from build123d import *

# Parameters (mm, degrees)
EXTRUDE_DEPTH     = 20
BOX003_W          = 15
BOX003_H          = 7.5
BOX003_DEPTH      = 6
CYLINDER003_R     = 2.1
CYLINDER003_DEPTH = 5
CYLINDER002_R     = 1.05
CYLINDER002_DEPTH = 7
BOX002_W          = 13
BOX002_H          = 13
BOX002_DEPTH      = 6
CYLINDER001_R     = 2.65
CYLINDER001_DEPTH = 5
CYLINDER_R        = 5.2
CYLINDER_DEPTH    = 20
BOX001_W          = 20.5
BOX001_H          = 20.5
BOX001_DEPTH      = 25
BOX004_W          = 7.5
BOX004_H          = 13
BOX004_DEPTH      = 6
BOX_W             = 40.5
BOX_H             = 62.8
BOX_DEPTH         = 25
FILLET_1_R        = 3
FILLET_2_R        = 1


with BuildPart() as obj1:
    # Sketch → Extrude (new body)
    with BuildSketch(Plane.YZ):
        with BuildLine():
            ThreePointArc((-3.606243, 3.606246), (0, -5.1), (3.606243, 3.606246))
            Line((2.112489, 5.1), (3.606243, 3.606246))
            Line((-2.112489, 5.1), (2.112489, 5.1))
            Line((-3.606243, 3.606246), (-2.112489, 5.1))
        make_face()
    extrude(amount=EXTRUDE_DEPTH)


with BuildPart() as obj1_1:
    # Extrude placement: moved
    add(obj1.part.moved(Location((20.5, 41.65, 15))))


with BuildPart() as hueco_taladro4:
    # Box003 → Box003 (new body)
    with BuildSketch(Plane(origin=(0, 39, 14), x_dir=(1, 0, 0), z_dir=(0, 0, 1))):
        with Locations((7.5, 3.75)):
            Rectangle(BOX003_W, BOX003_H)
    extrude(amount=BOX003_DEPTH)


with BuildPart() as taladro4:
    # Cylinder003 → Cylinder003 (new body)
    with BuildSketch(Plane(origin=(10, 42.7, 20), x_dir=(1, 0, 0), z_dir=(0, 0, 1))):
        Circle(CYLINDER003_R)
    extrude(amount=CYLINDER003_DEPTH)


with BuildPart() as clone005:
    # Clone005 base: copy of taladro4
    add(taladro4.part)


with BuildPart() as clone005_1:
    # Clone005 placement: moved
    add(clone005.part.moved(Location((15.5, 13.1, 0))))


with BuildPart() as taladro_endstop:
    # Cylinder002 → Cylinder002 (new body)
    with BuildSketch(Plane(origin=(35.5, 26.14, 12), x_dir=(1, 0, 0), z_dir=(0, 0, 1))):
        Circle(CYLINDER002_R)
    extrude(amount=CYLINDER002_DEPTH)


with BuildPart() as clone004:
    # Clone004 base: copy of taladro_endstop
    add(taladro_endstop.part)


with BuildPart() as clone004_1:
    # Clone004 placement: moved
    add(clone004.part.moved(Location((0, 7, 0))))


with BuildPart() as hueco_endstop:
    # Box002 → Box002 (new body)
    with BuildSketch(Plane(origin=(27.5, 23.14, 19), x_dir=(1, 0, 0), z_dir=(0, 0, 1))):
        with Locations((6.5, 6.5)):
            Rectangle(BOX002_W, BOX002_H)
    extrude(amount=BOX002_DEPTH)


with BuildPart() as taladro5:
    # Cylinder001 → Cylinder001 (new body)
    with BuildSketch(Plane(origin=(30.5, 10, 0), x_dir=(1, 0, 0), z_dir=(0, 0, 1))):
        Circle(CYLINDER001_R)
    extrude(amount=CYLINDER001_DEPTH)


with BuildPart() as clone002:
    # Clone002 base: copy of taladro5
    add(taladro5.part)


with BuildPart() as clone002_1:
    # Clone002 placement: moved
    add(clone002.part.moved(Location((-20.5, 21, 0))))


with BuildPart() as clone003:
    # Clone003 base: copy of Clone002
    add(clone002_1.part)


with BuildPart() as clone003_1:
    # Clone003 placement: moved
    add(clone003.part.moved(Location((0, 21.3, 0))))


with BuildPart() as taladro10:
    # Cylinder → Cylinder (new body)
    with BuildSketch(Plane(origin=(30.5, 10, 5), x_dir=(1, 0, 0), z_dir=(0, 0, 1))):
        Circle(CYLINDER_R)
    extrude(amount=CYLINDER_DEPTH)


with BuildPart() as clone:
    # Clone base: copy of taladro10
    add(taladro10.part)


with BuildPart() as clone_1:
    # Clone placement: moved
    add(clone.part.moved(Location((-20.5, 21, 0))))


with BuildPart() as clone001:
    # Clone001 base: copy of Clone
    add(clone_1.part)


with BuildPart() as clone001_1:
    # Clone001 placement: moved
    add(clone001.part.moved(Location((0, 21.3, 0))))


with BuildPart() as obj2:
    # Box001 → Box001 (new body)
    with BuildSketch(Plane.XY):
        with Locations((10.25, 10.25)):
            Rectangle(BOX001_W, BOX001_H)
    extrude(amount=BOX001_DEPTH)


with BuildPart() as huecos:
    # Box004 → Box004 (new body)
    with BuildSketch(Plane(origin=(21.75, 49.8, 14), x_dir=(1, 0, 0), z_dir=(0, 0, 1))):
        with Locations((3.75, 6.5)):
            Rectangle(BOX004_W, BOX004_H)
    extrude(amount=BOX004_DEPTH)

    # Fusion: union hueco_taladro4, Clone005, taladro4, Clone004, taladro_endstop, hueco_endstop, Clone003, Clone002, taladro5, Clone001, Clone, taladro10, obj2
    add(hueco_taladro4.part)
    add(clone005_1.part)
    add(taladro4.part)
    add(clone004_1.part)
    add(taladro_endstop.part)
    add(hueco_endstop.part)
    add(clone003_1.part)
    add(clone002_1.part)
    add(taladro5.part)
    add(clone001_1.part)
    add(clone_1.part)
    add(taladro10.part)
    add(obj2.part)


with BuildPart() as obj3:
    # Box → Box (new body)
    with BuildSketch(Plane.XY):
        with Locations((20.25, 31.4)):
            Rectangle(BOX_W, BOX_H)
    extrude(amount=BOX_DEPTH)

    # Cut: cut huecos
    add(huecos.part, mode=Mode.SUBTRACT)

    # Cut001: cut obj1
    add(obj1_1.part, mode=Mode.SUBTRACT)

    # Fillet 1
    fillet_1_edges = [obj3.edges().sort_by_distance(p)[0] for p in [
        (0, 62.8, 12.5),
        (40.5, 62.8, 12.5),
        (40.5, 0, 12.5),
    ]]
    fillet(fillet_1_edges, radius=FILLET_1_R)

    # Fillet 2
    fillet_2_edges = [obj3.edges().sort_by_distance(p)[0] for p in [
        (0, 20.5, 12.5),
        (20.5, 0, 12.5),
    ]]
    fillet(fillet_2_edges, radius=FILLET_2_R)


with BuildPart() as obj4:
    # Part__Mirroring: instance of obj3
    add(obj3.part.mirror(Plane(origin=(0, 0, 0), x_dir=(1, 0, 0), z_dir=(0, 1, 0))))


solid = obj4.part
The model under review builds one solid part; all positions refer to its coordinate system, in mm. A direction names the side the tool comes from. Round coordinates to 2 decimals unless told otherwise and drop trailing zeros. Write each loop counter-clockwise with the first axis right and the second up, starting at its lowest first coordinate (ties: lowest second). Pieces come first, ordered by that corner, then holes. Notation, with made-up numbers: (-13, 64) - (13, 64) arc R35 cw to (13, 99) - close; hole circle Ø8 at (47.25, -21). An arc over 180 degrees is marked (long way). One line per item, written item: value. Start each with the question number.
1. The part is to be moulded in two halves that separate along Z. For faces 1 (the face through (15, -43, 17)), 2 (the face through (9, -55, 5)), 3 (the face through (0.86, -61.9, 12.68)), say which applies: released by +Z, released by -Z, zero draft, split by the parting line, or undercut.
2. To check wall thickness, follow L1, parallel to X at y = -10, z = 16.75; L2, parallel to Y at x = 11, z = 8.5; L3, parallel to X at y = -52, z = 8.5. State the ranges of each line that lie inside material, in increasing order. Write a range as from..to.
3. Consider section B-B on z = 15. Write out the cut boundary in (x, y).
4. Consider section C-C on x = 10. Write out the cut boundary in (y, z).
5. Consider section D-D on z = 11. Write out the cut boundary in (x, y), and give its area (3 significant figures).
6. Clearance check with flat-ended pins moving along their axes: P1, Ø1.8, axis at y = -32.5, z = 21, coming from the +X side; P2, Ø6, axis at x = 10, y = -52.3, coming from the +Z side; P3, Ø0.6, axis at x = 35.5, y = -26, coming from the +Z side. State where each tip first meets the part, or that it passes through.
7. Machinability: for faces 4 (the face through (30, -42, 20.1)), 5 (the face through (25, -56, 14)), 6 (the face through (9.54, -40.65, 22.46)), which of the approach directions +Z, -Z, +X, -X, +Y, -Y give a long, thin tool a straight path to every point of the face, cutting with its end or side? Answer none if there is none.
8. Consider section A-A on y = -10. Write out the cut boundary in (x, z), and give its area (4 significant figures).
Checks:
1. face 1: undercut
1. face 2: released by +Z
1. face 3: zero draft
2. L1: x = 20.5..25.3, 35.7..40.5
2. L2: y = -62.8..-57.4, -47.2..-36.1, -25.9..-20.5
2. L3: x = 0..4.81, 15.19..40.5
3. outline: (0, -59.8) arc R3 ccw to (3, -62.8) - (21.75, -62.8) - (21.75, -49.8) - (29.25, -49.8) - (29.25, -62.8) - (37.5, -62.8) arc R3 ccw to (40.5, -59.8) - (40.5, -46.75) - (20.5, -46.75) - (20.5, -36.55) - (40.5, -36.55) - (40.5, -3) arc R3 ccw to (37.5, 0) - (21.5, 0) arc R1 ccw to (20.5, -1) - (20.5, -20.5) - (1, -20.5) arc R1 ccw to (0, -21.5) - (0, -39) - (15, -39) - (15, -46.5) - (0, -46.5) - close; hole circle Ø10.4 at (10, -52.3); hole circle Ø10.4 at (10, -31); hole circle Ø10.4 at (30.5, -10); hole circle Ø2.1 at (35.5, -33.14); hole circle Ø2.1 at (35.5, -26.14)
4. outline: (-62.8, 0) - (-54.95, 0) - (-54.95, 5) - (-57.5, 5) - (-57.5, 25) - (-62.8, 25) - close; (-49.65, 0) - (-33.65, 0) - (-33.65, 5) - (-36.2, 5) - (-36.2, 25) - (-40.6, 25) - (-40.6, 20) - (-39, 20) - (-39, 14) - (-46.5, 14) - (-46.5, 20) - (-44.8, 20) - (-44.8, 25) - (-47.1, 25) - (-47.1, 5) - (-49.65, 5) - close; (-28.35, 0) - (-20.5, 0) - (-20.5, 25) - (-25.8, 25) - (-25.8, 5) - (-28.35, 5) - close
5. outline: (0, -59.8) arc R3 ccw to (3, -62.8) - (37.5, -62.8) arc R3 ccw to (40.5, -59.8) - (40.5, -44.81) - (20.5, -44.81) - (20.5, -38.49) - (40.5, -38.49) - (40.5, -3) arc R3 ccw to (37.5, 0) - (21.5, 0) arc R1 ccw to (20.5, -1) - (20.5, -20.5) - (1, -20.5) arc R1 ccw to (0, -21.5) - close; hole circle Ø10.4 at (10, -52.3); hole circle Ø10.4 at (10, -31); hole circle Ø10.4 at (30.5, -10)
5. area: 1,740 mm^2
6. P1: stops at x = 27.5
6. P2: stops at z = 5
6. P3: stops at z = 12
7. face 4: +X
7. face 5: -Y
7. face 6: +Z
8. outline: (20.5, 0) - (27.85, 0) - (27.85, 5) - (25.3, 5) - (25.3, 25) - (20.5, 25) - close; (33.15, 0) - (40.5, 0) - (40.5, 25) - (35.7, 25) - (35.7, 5) - (33.15, 5) - close
8. area: 265.5 mm^2
